```python
from build123d import *

# Parameters (mm, degrees)
SKETCH1_R             = 11.43
SKETCH1_R_2           = 5.08
BOSS_EXTRUDE1_DEPTH   = 3.175
FILLET1_R             = 0.635
F_2_56_TAPPED_HOLE1_D = 1.778


with BuildPart() as part:
    # Sketch1 → Boss-Extrude1 (new body)
    with BuildSketch(Plane.XY):
        Circle(SKETCH1_R)
        Circle(SKETCH1_R_2, mode=Mode.SUBTRACT)
    extrude(amount=BOSS_EXTRUDE1_DEPTH)

    # Fillet1
    fillet1_edges = [part.edges().sort_by_distance(p)[0] for p in [
        (-5.08, 0, 0),
        (-5.08, 0, 3.175),
    ]]
    fillet(fillet1_edges, radius=FILLET1_R)

    # #2-56 Tapped Hole1 (through all)
    with Locations(Plane.XY.offset(3.175)):
        with Locations((0, 9.525)):
            f_2_56_tapped_hole1 = Hole(F_2_56_TAPPED_HOLE1_D / 2)

    # Mirror1: #2-56 Tapped Hole1 across plane
    add(f_2_56_tapped_hole1.mirror(Plane.ZX), mode=Mode.SUBTRACT)


solid = part.part
```
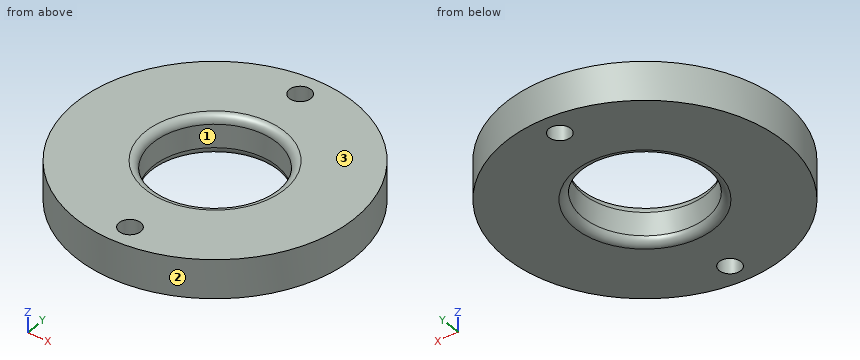
Build history of the part. All positions in model axes, mm. Face numbers are marked on the shaded views. Round coordinates to 2 decimals unless told otherwise and drop trailing zeros. Write each loop counter-clockwise with the first axis right and the second up, starting at its lowest first coordinate (ties: lowest second). Pieces come first, ordered by that corner, then holes.
1) Drill centre lines: probe 1 along Y at (x, z) = (0, 1.95); probe 2 along X at (y, z) = (-1.25, 1.6); probe 3 along Y at (x, z) = (-2.75, 0.6). Where is each one in solid material? Low to high.
2) Band-saw the part on D-D, the plane y = 10. List the corners of the cut face in (x, z) (3 decimals), and give its area (3 significant figures).
3) Mould opens along X. For the marked faces 1, 2 and 3 say: +X half, -X half, draft (parallel to the pull), parting line (faces both ways), or undercut.
4) Band-saw the part on A-A, the plane x = 0. List the corners of the cut face in (y, z) (3 decimals).
5) Pin check, flat tip, straight feed: pin 1 (1.5 mm diameter, centred on x = 7, z = 2.5, fed in from -Y). Stop position of the tip, or through.
6) Band-saw the part on C-C, the plane z = 2.85. List the corners of the cut face in (x, y) (3 decimals), and give its area (3 significant figures).
7) Band-saw the part on B-B, the plane y = 0. List the corners of the cut face in (x, z) (3 decimals).
Ans:
1. probe 1: y = -11.43 to -10.41, -8.64 to -5.08, 5.08 to 8.64, 10.41 to 11.43
1. probe 2: x = -11.36 to -4.92, 4.92 to 11.36
1. probe 3: y = -11.09 to -4.27, 4.27 to 11.09
2. outline: (-5.536, 0) - (-0.751, 0) - (-0.751, 3.175) - (-5.536, 3.175) - close; (0.751, 0) - (5.536, 0) - (5.536, 3.175) - (0.751, 3.175) - close
2. area: 30.4 mm2
3. face 1: undercut
3. face 2: parting line
3. face 3: draft
4. outline: (-11.43, 0) - (-10.414, 0) - (-10.414, 3.175) - (-11.43, 3.175) - close; (-8.636, 0) - (-5.715, 0) arc R0.635 ccw to (-5.08, 0.635) - (-5.08, 2.54) arc R0.635 ccw to (-5.715, 3.175) - (-8.636, 3.175) - close; (5.08, 0.635) arc R0.635 ccw to (5.715, 0) - (8.636, 0) - (8.636, 3.175) - (5.715, 3.175) arc R0.635 ccw to (5.08, 2.54) - close; (10.414, 0) - (11.43, 0) - (11.43, 3.175) - (10.414, 3.175) - close
5. pin 1: stops at y = -9.57
6. outline: circle Ø22.86 at (0, 0); hole circle Ø10.322 at (0, 0); hole circle Ø1.778 at (0, -9.525); hole circle Ø1.778 at (0, 9.525)
6. area: 322 mm2
7. outline: (-11.43, 0) - (-5.715, 0) arc R0.635 ccw to (-5.08, 0.635) - (-5.08, 2.54) arc R0.635 ccw to (-5.715, 3.175) - (-11.43, 3.175) - close; (5.08, 0.635) arc R0.635 ccw to (5.715, 0) - (11.43, 0) - (11.43, 3.175) - (5.715, 3.175) arc R0.635 ccw to (5.08, 2.54) - close
